CAD build for the part. Positions are in the model's coordinates, mm. A direction names the side the tool comes from. Round coordinates to 2 decimals unless told otherwise and drop trailing zeros. Order: outer loops, then holes, each group sorted by start corner. A loop starts at its lowest first (then second) coordinate and runs counter-clockwise, first axis right, second up. Notation, with made-up numbers: M 4,-33 L 55,-33 A15 cw 55,-12 Z; hole C -28.75,65.25 d7. An arc over 180 degrees is marked long. Answer as a JSON object with one key per item and string values.
```python
from build123d import *

# Parameters (mm, degrees)
BOSS_EXTRUDE1_DEPTH     = 38.1
CUT_EXTRUDE2_DEPTH      = 18.9865
CUT_EXTRUDE4_DEPTH      = 3.0193
CUT_EXTRUDE4_DEPTH_BACK = 2.5367
FILLET3_R               = 5.08
SKETCH8_R               = 2.85115
CUT_EXTRUDE5_DEPTH      = 3.0193
CUT_EXTRUDE5_DEPTH_BACK = 2.5367
CHAMFER1_SIZE           = 0.254


with BuildPart() as part:
    # Sketch1 → Boss-Extrude1 (new body)
    with BuildSketch(Plane(origin=(0, 0, 0), x_dir=(1, 0, 0), z_dir=(0, 1, 0))):
        Polygon((9.770109876, 2.0193), (6.989445062, 0), (-6.989445062, 0), (-9.770109876, 2.0193), (-23.749, 2.0193), (-23.749, 3.556), (-9.271, 3.556), (-6.490335186, 1.5367), (6.490335186, 1.5367), (9.271, 3.556), (23.749, 3.556), (23.749, 2.0193), align=None)
    extrude(amount=BOSS_EXTRUDE1_DEPTH)

    # Sketch3 → Cut-Extrude2 (cut)
    with BuildSketch(Plane(origin=(0, 38.1, 0), x_dir=(1, 0, 0), z_dir=(0, 1, 0))):
        Polygon((-9.770109876, 3.91845022), (-9.770109876, 2.0193), (-6.490335186, -0.36245022), (-6.490335186, 1.5367), align=None)
        Polygon((6.490335186, 1.5367), (9.770109876, 3.91845022), (9.770109876, 2.0193), (6.490335186, -0.36245022), align=None)
    extrude(amount=-CUT_EXTRUDE2_DEPTH, mode=Mode.SUBTRACT)

    # Sketch6 → Cut-Extrude4 (cut, two sides)
    with BuildSketch(Plane(origin=(0, 0, -1.5367), x_dir=(-1, 0, 0), z_dir=(0, 0, -1))) as cut_extrude4_sk:
        with BuildLine():
            Line((-6.490335186, 26.123264814), (-8.408477538, 26.123264814))
            Line((-8.408477538, 26.123264814), (-8.408477538, 40.625106564))
            Line((-8.408477538, 40.625106564), (8.313468388, 40.625106564))
            Line((8.313468388, 40.625106564), (8.313468388, 26.123264814))
            Line((8.313468388, 26.123264814), (6.490335186, 26.123264814))
            ThreePointArc((6.490335186, 26.123264814), (0, 32.6136), (-6.490335186, 26.123264814))
        make_face()
    extrude(amount=CUT_EXTRUDE4_DEPTH, mode=Mode.SUBTRACT)
    extrude(cut_extrude4_sk.sketch, amount=-CUT_EXTRUDE4_DEPTH_BACK, mode=Mode.SUBTRACT)

    # Fillet3
    fillet3_edges = [part.edges().sort_by_distance(p)[0] for p in [
        (-9.770109876, 38.1, -2.78765),
        (9.770109876, 38.1, -2.78765),
    ]]
    fillet(fillet3_edges, radius=FILLET3_R)

    # Sketch8 → Cut-Extrude5 (cut, two sides)
    with BuildSketch(Plane.XY.offset(-2.0193)) as cut_extrude5_sk:
        with Locations((-16.32585, 31.33725)):
            Circle(SKETCH8_R)
        with Locations((-16.32585, 6.76275)):
            Circle(SKETCH8_R)
        with Locations((16.32585, 6.76275)):
            Circle(SKETCH8_R)
        with Locations((16.32585, 31.33725)):
            Circle(SKETCH8_R)
    extrude(amount=CUT_EXTRUDE5_DEPTH, mode=Mode.SUBTRACT)
    extrude(cut_extrude5_sk.sketch, amount=-CUT_EXTRUDE5_DEPTH_BACK, mode=Mode.SUBTRACT)

    # Chamfer1
    chamfer1_edges = [part.edges().sort_by_distance(p)[0] for p in [
        (-19.177, 31.33725, -2.0193),
        (-19.177, 6.76275, -2.0193),
        (13.4747, 6.76275, -2.0193),
        (13.4747, 31.33725, -2.0193),
    ]]
    chamfer(chamfer1_edges, length=CHAMFER1_SIZE)


solid = part.part
```
Item 1: Wall check: line 1 along X through (y, z) = (28, -3); line 2 along Z through (x, y) = (15, 35.5); line 3 along Z through (x, y) = (4, 11). Give the ranges that are in metal, low to high. Write a range as [from, to].
Worked answers:
{"line 1": "x = [-23.75, -9.77], [9.77, 23.75]", "line 2": "z = [-3.56, -2.02]", "line 3": "z = [-1.54, 0]"}
Item 2: Drop flat-ended pins along their axis: pin 1 Ø7 at (x, y) = (-15.5, 13.5) entering from +Z; pin 2 Ø0.5 at (y, z) = (22.5, -0.5) entering from -X; pin 3 Ø1.5 at (x, y) = (-18, 32) entering from +Z; pin 4 Ø0.5 at (y, z) = (24, -0.5) entering from +X. Give the stop position or say it passes through.
Worked answers:
{"pin 1": "stops at z = -2.02", "pin 2": "stops at x = -6.49", "pin 3": "passes through", "pin 4": "stops at x = 6.49"}
Item 3: 3-axis set-ups, long thin cutter, end or side, ignore diameter. For faces 1 (the flat face through (17, 19, -2.019)), 2 (the flat face through (0, 16, -1.537)), 3 (the flat face through (8, 19.114, -2)): which of +Z, -Z, +X, -X, +Y, -Y reach the whole face in a straight line?
Worked answers:
{"face 1": "+Z, +X, +Y, -Y", "face 2": "-Z, +Y, -Y", "face 3": "+Z, -Z, +Y"}
Item 4: Saw through at A-A on y = 35. List the corners of the cut face in (x, z).
Worked answers:
{"outline": "M -23.75,-3.56 L -10.17,-3.56 L -10.17,-2.02 L -23.75,-2.02 Z; M 10.17,-3.56 L 23.75,-3.56 L 23.75,-2.02 L 10.17,-2.02 Z"}
Item 5: Saw through at C-C on y = 13.5. List the corners of the cut face in (x, z).
Worked answers:
{"outline": "M -23.75,-3.56 L -9.27,-3.56 L -6.49,-1.54 L 6.49,-1.54 L 9.27,-3.56 L 23.75,-3.56 L 23.75,-2.02 L 9.77,-2.02 L 6.99,0 L -6.99,0 L -9.77,-2.02 L -23.75,-2.02 Z"}
Item 6: Saw through at D-D on z = -0.65. List the corners of the cut face in (x, y), and give its area (3 significant figures).
Worked answers:
{"outline": "M -7.88,0 L 7.88,0 L 7.88,19.11 L 6.49,19.11 L 6.49,26.12 A6.49 ccw -6.49,26.12 L -6.49,19.11 L -7.88,19.11 Z", "area": "459 mm2"}
Item 7: Saw through at B-B on x = 20. List the corners of the cut face in (y, z).
Worked answers:
{"outline": "M 0,-3.56 L 38.1,-3.56 L 38.1,-2.02 L 0,-2.02 Z"}
Item 8: Two-plate mould, pull along X, no slides. Class faces 4 (the flat face through (-19, 38.1, -3)), 5 (the cylindrical face through (14.06, 5.03, -2.91)), 6 (the cylindrical face through (-0.143, 32.612, -0.779)): released by +X, released by -X, zero draft, split by the parting line, or undercut.
Worked answers:
{"face 4": "zero draft", "face 5": "undercut", "face 6": "split by the parting line"}
